Here's the drawing with two shaded views (mm, measured from the low corner). I have some questions. A direction names the side the tool comes from. Coordinates: 2 decimals unless noted, no trailing zeros. Write each loop counter-clockwise with the first axis right and the second up, starting at its lowest first coordinate (ties: lowest second). Pieces come first, ordered by that corner, then holes.
Item 1: I want a section at B-B on x = 37. Please give me the cut outline in (y, z), then the cut area to 3 significant figures.
Item 2: If I drill on probe 1 along X at (y, z) = (18, 7); probe 2 along Y at (x, z) = (37, 1.5); probe 3 along X at (y, z) = (24.5, 0.5), over which ranges is the centre line in solid material (lowest first)?
Item 3: I want a section at D-D on x = 14. Please give me the cut outline in (y, z), then the cut area to 3 significant figures.
Item 4: I want a section at C-C on z = 5. State how many separate pieces and enclosed holes the cut face has, then the cut area to 3 significant figures.
Item 5: I want a section at A-A on y = 29. Please give me the cut outline in (x, z), then the cut area to 3 significant figures.
Item 6: Which directions (+Z, -Z, +X, -X, +Y, -Y) give clear straight access to the entire face, cutting with the end or side of a thin tool? Please do the marked faces 4, 5, 6, 7 and 8.
Item 7: Thinking about a two-plate mould opening in X: for the marked faces 1, 2 and 3, which applies, +X half, -X half, draft (parallel to the pull), parting line (faces both ways), or undercut?
Item 8: For P1, Ø6, axis at y = 21.5, z = 6, coming from the -X side; P2, Ø2.5, axis at x = 5, z = 5, coming from the +Y side; P3, Ø2.5, axis at y = 26.5, z = 5, coming from the -X side; P4, Ø4, axis at y = 6.5, z = 4, coming from the +X side, each with a flat end and sliding along its axis, tell me the tip position at first contact or that it passes through.
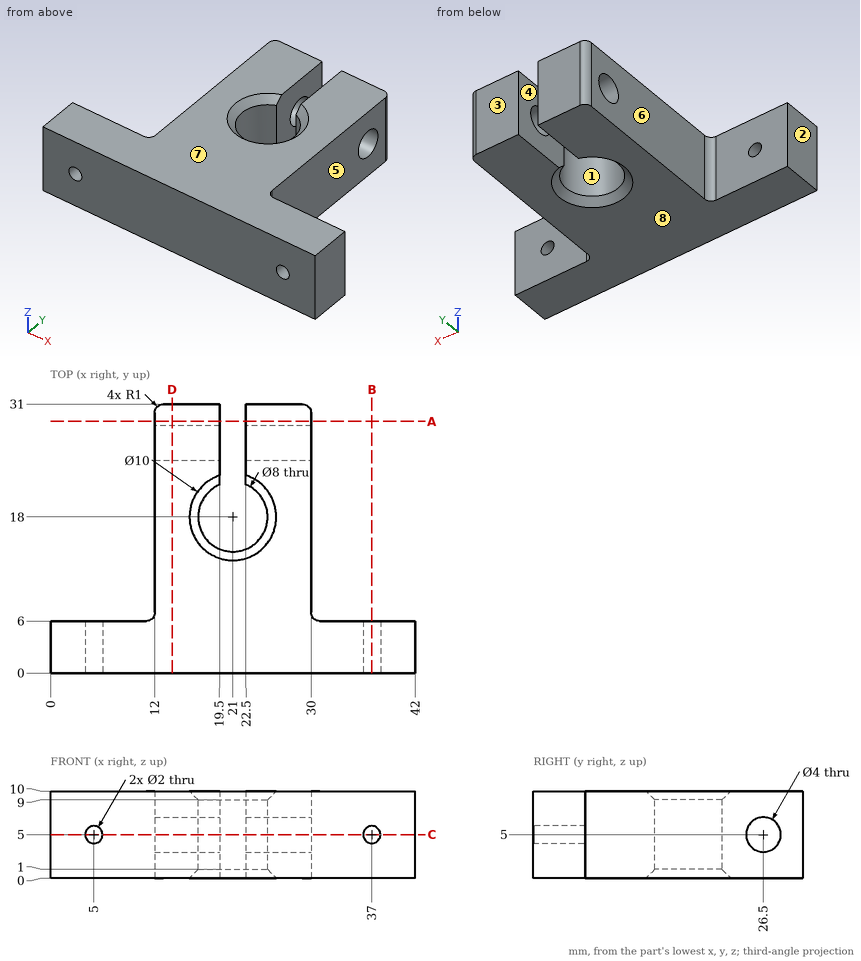
Response values:
1. outline: (0, 0) - (6, 0) - (6, 4) - (0, 4) - close; (0, 6) - (6, 6) - (6, 10) - (0, 10) - close
1. area: 48.0 mm2
2. probe 1: x = 12 to 17, 25 to 30
2. probe 2: y = 0 to 6
2. probe 3: x = 12 to 19.5, 22.5 to 30
3. outline: (0, 0) - (31, 0) - (31, 10) - (0, 10) - close; hole circle Ø4 at (26.5, 5)
3. area: 297 mm2
4. separate pieces: 5
4. enclosed holes: 0
4. area: 540 mm2
5. outline: (12, 0) - (19.5, 0) - (19.5, 10) - (12, 10) - close; (22.5, 0) - (30, 0) - (30, 10) - (22.5, 10) - close
5. area: 150 mm2
6. face 4: +Z, -Z, +Y
6. face 5: +Z, -Z, +X, +Y
6. face 6: +Z, -Z, -X, +Y
6. face 7: +Z, +X, -X, +Y, -Y
6. face 8: -Z, +X, -X, +Y, -Y
7. face 1: undercut
7. face 2: -X half
7. face 3: draft
8. P1: stops at x = 12
8. P2: stops at y = 6
8. P3: passes through
8. P4: stops at x = 42
